from build123d import *

# Parameters (mm, degrees)
F0_W     = 37.084
F0_H     = 37.084
F1_DEPTH = 101.6
F2_W     = 26.924
F2_H     = 26.924
F3_DEPTH = 50.8
F4_R     = 3.175
F5_DEPTH = 37.085
F6_R     = 3.175
F7_DEPTH = 37.085


with BuildPart() as f1:
    # F0 (on Top) → F1 (new body)
    with BuildSketch(Plane.XY):
        Rectangle(F0_W, F0_H)
    extrude(amount=F1_DEPTH)

    # F2 (on face) → F3 (cut)
    with BuildSketch(Plane(origin=(0, 0, 0), x_dir=(1, 0, 0), z_dir=(0, 0, -1))):
        Rectangle(F2_W, F2_H)
    extrude(amount=-F3_DEPTH, mode=Mode.SUBTRACT)

    # F4 (on face) → F5 (cut, through all)
    with BuildSketch(Plane.XZ.offset(18.542)):
        with Locations((0, 12.7)):
            Circle(F4_R)
    extrude(amount=-F5_DEPTH, mode=Mode.SUBTRACT)

    # F6 (on face) → F7 (cut, through all)
    with BuildSketch(Plane.XZ.offset(18.542)):
        with Locations((0, 38.1)):
            Circle(F6_R)
    extrude(amount=-F7_DEPTH, mode=Mode.SUBTRACT)


solid = f1.part
Input: part model. Units: mm. Frame: model coordinates. A direction names the side the tool comes from. Round coordinates to 2 decimals unless told otherwise and drop trailing zeros. Order: outer loops, then holes, each group sorted by start corner. A loop starts at its lowest first (then second) coordinate and runs counter-clockwise, first axis right, second up. Notation, with made-up numbers: (2.25, 22) - (52.25, 22) arc R24 cw to (52.25, 50) - close; hole circle Ø3 at (18, -25). An arc over 180 degrees is marked (long way). Answer as a JSON object with one key per item and string values. Group by question number.
(1) Cut plane C-C (y = 6.5). Return loops of the section in (x, z), then the cut area to 3 significant figures.
(2) Cut plane D-D (z = 32). Return loops of the section in (x, y).
(3) Reachability of faces 1 (the face through (1.5, 16, 9.9)), 2 (the face through (0, 0, 50.8)) from +Z, -Z, +X, -X, +Y, -Y: full face, straight path, thin tool, end or side. Return the list, or none.
(4) Cut plane B-B (z = 12.7). Return loops of the section in (x, y) (3 decimals).
(5) Material intervals for probe 1 along Z at (x, y) = (0, -14.85) (3 decimals); probe 2 along Y at (x, z) = (4.5, 14); probe 3 along X at (y, z) = (15, 38), sorted ascending. Write a range as from..to.
(6) Draft query along Z for faces 3 (the face through (-18.542, 0, 50)), 4 (the face through (-0.69, -16.04, 35)), 5 (the face through (-17, 0, 0)). Return one class per face: released by +Z, released by -Z, zero draft, split by the parting line, or undercut.
(7) Pin query (flat end, axial travel): P1, Ø12, axis at x = 3.5, y = 0, coming from the -Z side. Return the tip coordinate at first contact, or that it passes through.
(8) Cut plane A-A (x = 0). Return loops of the section in (y, z) (3 decimals).
Here are the results:
{
 "1": {"outline": "(-18.54, 0) - (-13.46, 0) - (-13.46, 50.8) - (13.46, 50.8) - (13.46, 0) - (18.54, 0) - (18.54, 101.6) - (-18.54, 101.6) - close", "area": "2,400 mm^2"},
 "2": {"outline": "(-18.54, -18.54) - (18.54, -18.54) - (18.54, 18.54) - (-18.54, 18.54) - close; hole (-13.46, -13.46) - (13.46, -13.46) - (13.46, 13.46) - (-13.46, 13.46) - close"},
 "3": {"face 1": "+Y, -Y", "face 2": "-Z"},
 "4": {"outline": "(-18.542, -18.542) - (-3.175, -18.542) - (-3.175, -13.462) - (-13.462, -13.462) - (-13.462, 13.462) - (-3.175, 13.462) - (-3.175, 18.542) - (-18.542, 18.542) - close; (3.175, -18.542) - (18.542, -18.542) - (18.542, 18.542) - (3.175, 18.542) - (3.175, 13.462) - (13.462, 13.462) - (13.462, -13.462) - (3.175, -13.462) - close"},
 "5": {"probe 1": "z = 0..9.525, 15.875..34.925, 41.275..101.6", "probe 2": "y = -18.54..-13.46, 13.46..18.54", "probe 3": "x = -18.54..-3.17, 3.17..18.54"},
 "6": {"face 3": "zero draft", "face 4": "undercut", "face 5": "released by -Z"},
 "7": {"P1": "stops at z = 50.8"},
 "8": {"outline": "(-18.542, 0) - (-13.462, 0) - (-13.462, 9.525) - (-18.542, 9.525) - close; (-18.542, 15.875) - (-13.462, 15.875) - (-13.462, 34.925) - (-18.542, 34.925) - close; (-18.542, 41.275) - (-13.462, 41.275) - (-13.462, 50.8) - (13.462, 50.8) - (13.462, 41.275) - (18.542, 41.275) - (18.542, 101.6) - (-18.542, 101.6) - close; (13.462, 0) - (18.542, 0) - (18.542, 9.525) - (13.462, 9.525) - close; (13.462, 15.875) - (18.542, 15.875) - (18.542, 34.925) - (13.462, 34.925) - close"}
}
